Build history of the part. All positions in model axes, mm. A direction names the side the tool comes from. Round coordinates to 2 decimals unless told otherwise and drop trailing zeros. Write each loop counter-clockwise with the first axis right and the second up, starting at its lowest first coordinate (ties: lowest second). Pieces come first, ordered by that corner, then holes.
from build123d import *

# Parameters (mm, degrees)
BOSS_EXTRUDE_BASE_DEPTH = 6
SKETCH4_W               = 1.75
SKETCH4_H               = 40
CUT_EXTRUDE_SLOT_DEPTH  = 4.5


with BuildPart() as part:
    # Sketch1 → Boss-Extrude-Base (new body)
    with BuildSketch(Plane.XY):
        with BuildLine():
            Line((10.072988134, 10.472135955), (10.072988134, 46.527864045))
            ThreePointArc((10.072988134, 46.527864045), (13.45569569, 45.031838638), (17.072988134, 45.803847577))
            ThreePointArc((17.072988134, 45.803847577), (17.439013538, 47.169872981), (16.072988134, 47.535898385))
            ThreePointArc((16.072988134, 47.535898385), (10.072988134, 51), (16.072988134, 54.464101615))
            ThreePointArc((16.072988134, 54.464101615), (17.439013538, 54.830127019), (17.072988134, 56.196152423))
            ThreePointArc((17.072988134, 56.196152423), (13.45569569, 56.968161362), (10.072988134, 55.472135955))
            Line((10.072988134, 55.472135955), (10.072988134, 61.375))
            Line((10.072988134, 61.375), (0.072988134, 61.375))
            Line((0.072988134, 61.375), (0.072988134, 10))
            ThreePointArc((0.072988134, 10), (3.001920322, 2.928932188), (10.072988134, 0))
            Line((10.072988134, 0), (14.072988134, 0))
            ThreePointArc((14.072988134, 0), (15.625902405, 0.204445042), (17.072988134, 0.803847577))
            ThreePointArc((17.072988134, 0.803847577), (17.439013538, 2.169872981), (16.072988134, 2.535898385))
            ThreePointArc((16.072988134, 2.535898385), (10.072988134, 6), (16.072988134, 9.464101615))
            ThreePointArc((16.072988134, 9.464101615), (17.439013538, 9.830127019), (17.072988134, 11.196152423))
            ThreePointArc((17.072988134, 11.196152423), (13.45569569, 11.968161362), (10.072988134, 10.472135955))
        make_face()
    extrude(amount=BOSS_EXTRUDE_BASE_DEPTH)

    # Sketch4 → Cut-Extrude-Slot (cut)
    with BuildSketch(Plane.XY.offset(6)):
        with Locations((3.947988134, 38.5)):
            Rectangle(SKETCH4_W, SKETCH4_H)
    extrude(amount=-CUT_EXTRUDE_SLOT_DEPTH, mode=Mode.SUBTRACT)


solid = part.part
1) Which spindle directions (+Z, -Z, +X, -X, +Y, -Y) get a long thin tool onto all of the face, cutting with end or side? Do faces 5 (the flat face through (4, 39, 1.5)), 6 (the flat face through (10.073, 58, 3)), 7 (the flat face through (12, 0, 3)). Say none if no direction does.
Results:
face 5: +Z
face 6: +Z, -Z, +Y
face 7: +Z, -Z, +X, -X, -Y
2) Slice it at A-A (y = 51). Write the cut outline in (x, z).
Results:
outline: (0.07, 0) - (10.07, 0) - (10.07, 6) - (4.82, 6) - (4.82, 1.5) - (3.07, 1.5) - (3.07, 6) - (0.07, 6) - close
3) Wall check: L1, parallel to Y at x = 13.75, z = 0.4; L2, parallel to X at y = 25.5, z = 4.55; L3, parallel to Y at x = 12, z = 3.15. Give the ranges that are in metal, low to high.
Results:
L1: y = 0 to 2.01, 9.99 to 11.99, 45.01 to 47.01, 54.99 to 56.99
L2: x = 0.07 to 3.07, 4.82 to 10.07
L3: y = 0 to 2.58, 9.42 to 11.63, 45.37 to 47.58, 54.42 to 56.63
4) Mould opens along Y. For faces 1 (the flat face through (5, 61.375, 3)), 2 (the cylindrical face through (14, 12, 3)), 3 (the cylindrical face through (2.92, 3.01, 2.96)), 4 (the flat face through (0.073, 36, 3)) say: released by +Y, released by -Y, zero draft, split by the parting line, or undercut.
Results:
face 1: released by +Y
face 2: undercut
face 3: released by -Y
face 4: zero draft
5) Slice it at D-D (x = 13.25). Write the cut outline in (y, z), plus the area to 3 significant figures.
Results:
outline: (0, 0) - (2.09, 0) - (2.09, 6) - (0, 6) - close; (9.91, 0) - (11.94, 0) - (11.94, 6) - (9.91, 6) - close; (45.06, 0) - (47.09, 0) - (47.09, 6) - (45.06, 6) - close; (54.91, 0) - (56.94, 0) - (56.94, 6) - (54.91, 6) - close
area: 49.0 mm2
6) Pin check, flat tips, straight feed: pin 1 Ø1.5 at (x, z) = (15, 2.5) entering from -Y; pin 2 Ø3 at (y, z) = (59.5, 3.5) entering from +X; pin 3 Ø0.5 at (x, z) = (3.5, 3) entering from -Y. Stop position of each tip, or through.
Results:
pin 1: stops at y = 0
pin 2: stops at x = 10.07
pin 3: stops at y = 2.25
7) Slice it at C-C (z = 2.75). Write the cut outline in (x, y) (3 decimals), plus the area to 3 significant figures.
Results:
outline: (0.073, 10) arc R10 ccw to (10.073, 0) - (14.073, 0) arc R6 ccw to (17.073, 0.804) arc R1 ccw to (16.073, 2.536) arc R4 cw (long way) to (16.073, 9.464) arc R1 ccw to (17.073, 11.196) arc R6 ccw to (10.073, 10.472) - (10.073, 46.528) arc R6 ccw to (17.073, 45.804) arc R1 ccw to (16.073, 47.536) arc R4 cw (long way) to (16.073, 54.464) arc R1 ccw to (17.073, 56.196) arc R6 ccw to (10.073, 55.472) - (10.073, 61.375) - (0.073, 61.375) - close; hole (3.073, 18.5) - (4.823, 18.5) - (4.823, 58.5) - (3.073, 58.5) - close
area: 589 mm2
8) Slice it at B-B (x = 11). Write the cut outline in (y, z), plus the area to 3 significant figures.
Results:
outline: (0, 0) - (3.44, 0) - (3.44, 6) - (0, 6) - close; (8.56, 0) - (11.15, 0) - (11.15, 6) - (8.56, 6) - close; (45.85, 0) - (48.44, 0) - (48.44, 6) - (45.85, 6) - close; (53.56, 0) - (56.15, 0) - (56.15, 6) - (53.56, 6) - close
area: 67.3 mm2
